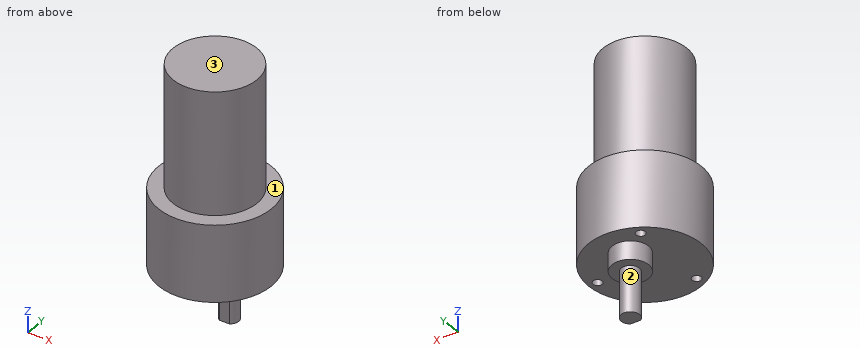
Autodesk Inventor part; units mm, degrees
ref_plane "作業平面1" through (0, 0, 0) normal (1, 0, 0) x (0, 0.3162, -0.9487)
ref_plane "YZ Plane" through (0, 0, 0) normal (1, 0, 0) x (0, 1, 0)
ref_plane "XZ Plane" through (0, 0, 0) normal (0, 1, 0) x (-1, 0, 0)
sketch "スケッチ1" plane through (0, 0, 0) normal (0, 0, 1) x (1, 0, 0)
  circle A0 centre (0, 0) radius 18.5
  dimension "d0" = 37
extrude "押し出し1" add sketch "スケッチ1" along normal blind 25
sketch "スケッチ2" plane through (0, 0, 25) normal (0, 0, 1) x (1, 0, 0)
  circle A0 centre (0, 0) radius 13.75
  dimension "d3" = 27.5
extrude "押し出し2" add sketch "スケッチ2" along normal blind 40
sketch "スケッチ3" plane through (0, 0, 0) normal (0, 0, -1) x (-1, 0, 0)
  circle A0 centre (0, 0) radius 18.5
  circle A1 centre (0, 7) radius 6
  dimension "d6" = 12
  dimension "d7" = 7
extrude "押し出し3" add sketch "スケッチ3" along normal blind 6 contours A1
sketch "スケッチ4" plane through (0, 7, -6) normal (0, 0, -1) x (-1, 0, 0)
  circle A0 centre (0, 0) radius 3
  point P0 (0, -7)
  dimension "d10" = 6
extrude "押し出し4" add sketch "スケッチ4" along normal blind 15
sketch "スケッチ5" plane through (0, 0, 0) normal (0, 0, -1) x (-1, 0, 0)
  circle A0 centre (0, 0) radius 18.5
  circle A1 centre (0, 0) radius 15.5
  line L0 (0, 0) -> (-15.5, 0)
  line L1 (7.75, 13.4234) -> (0, 0)
  line L2 (0, 0) -> (7.75, -13.4234)
  point P0 (-15.5, 0)
  point P1 (7.75, -13.4234)
  dimension "d13" = 31
  dimension "d14" = 120
  dimension "d15" = 120
hole "Hole1" at (15.5, 0, 0) at (-7.75, -13.4234, 0) at (-7.75, 13.4234, 0) direction (0, 0, 1) diameter 3 depth 3 tip angle 118
ref_plane "作業平面1" through (0, 0, 0) normal (1, 0, 0) x (0, 0.3162, -0.9487)
sketch "スケッチ6" plane through (0, 7, -21) normal (0, 0, -1) x (-1, 0, 0)
  arc A0 (-1.6583, -2.5) -> (1.6583, -2.5) centre (0, 0) ccw
  circle A1 centre (0, 0) radius 3
  line L0 (-1.6583, -2.5) -> (1.6583, -2.5)
  line L1 (0, 0) -> (-3, 0)
  point P0 (0, -7)
  dimension "d23" = 2.5
extrude "押し出し5" cut sketch "スケッチ6" against normal blind 12 contours L0 A0
properties part number "rs380ph_36"
Part model, mm, in its own coordinate system. Face numbers are marked on the shaded views. A direction names the side the tool comes from. Round coordinates to 2 decimals unless told otherwise and drop trailing zeros. Order: outer loops, then holes, each group sorted by start corner. A loop starts at its lowest first (then second) coordinate and runs counter-clockwise, first axis right, second up. Notation, with made-up numbers: M -20,46 L 38,46 A17 cw 38,78 Z; hole C 38,-7 d1. An arc over 180 degrees is marked long. Answer in a Markdown table with one row per item. Add a question column.
Q1. Wall check: L1, parallel to Y at x = -7.75, z = 0.7; L2, parallel to Z at x = -3, y = -16; L3, parallel to Z at x = -2, y = 12. Give the ranges that are in metal, low to high. Write a range as from..to.
Q2. Cut at D-D on y = -10. Give the cut face in (x, z), and give its area (3 significant figures).
Q3. Cut at C-C on z = -10.5. Give the cut face in (x, y).
Q4. Cut at B-B on y = 7. Give the cut face in (x, z).
Q5. Cut at A-A on x = 0. Give the cut face in (y, z).
Q6. Pin check, flat tips, straight feed: pin 1 (1 mm diameter, centred on x = 11, z = 10, fed in from +Y); pin 2 (5 mm diameter, centred on x = -7.75, y = 13.42, fed in from -Z); pin 3 (5 mm diameter, centred on x = 1, z = 15.5, fed in from -Y). Stop position of each tip, or through.
Q7. 3-axis set-ups, long thin cutter, end or side, ignore diameter. For the marked faces 1, 2 and 3: which of +Z, -Z, +X, -X, +Y, -Y reach the whole face in a straight line?
Established:
| question | item | result |
|---|---|---|
| 1 | L1 | y = -16.8..-14.92, -11.92..11.92, 14.92..16.8 |
| 1 | L2 | z = 0..25 |
| 1 | L3 | z = -6..65 |
| 2 | outline | M -15.56,0 L 15.56,0 L 15.56,25 L 9.44,25 L 9.44,65 L -9.44,65 L -9.44,25 L -15.56,25 Z |
| 2 | area | 1,530 mm2 |
| 3 | outline | M -1.66,4.5 L 1.66,4.5 A3 ccw long Z |
| 4 | outline | M -17.12,0 L -6,0 L -6,-6 L -3,-6 L -3,-21 L 3,-21 L 3,-6 L 6,-6 L 6,0 L 17.12,0 L 17.12,25 L 11.83,25 L 11.83,65 L -11.83,65 L -11.83,25 L -17.12,25 Z |
| 5 | outline | M -18.5,0 L 1,0 L 1,-6 L 4,-6 L 4,-9 L 4.5,-9 L 4.5,-21 L 10,-21 L 10,-6 L 13,-6 L 13,0 L 18.5,0 L 18.5,25 L 13.75,25 L 13.75,65 L -13.75,65 L -13.75,25 L -18.5,25 Z |
| 6 | pin 1 | stops at y = 15.23 |
| 6 | pin 2 | stops at z = 0 |
| 6 | pin 3 | stops at y = -18.5 |
| 7 | face 1 | +Z |
| 7 | face 2 | -Z |
| 7 | face 3 | +Z, +X, -X, +Y, -Y |
